from build123d import *


# Not quite as in the source:
# - a fillet or chamfer that OpenCascade refuses, or shapes differently, is made with other operations: its cross-section is extruded or revolved along the edge and cut away or added


with BuildPart() as f1:
    # F0 (on Front) → F1 (revolve)
    with BuildSketch(Plane.XZ):
        Polygon((-3.0760182999, 0), (0, 0), (0, 7.6753781177), (10.0012486801, 7.6753781177), (10.0012486801, 75.3582566977), (13.1937107071, 75.3582566977), (13.1937107071, 78.3602893353), (6.8093864247, 78.3602893353), (6.8093864247, 10.8100166544), (-3.0760182999, 10.8100166544), align=None)
    revolve(axis=Axis((-14.1970999539, 0, 39.5920351148), (0, 0, 1)))

    # F2: fillet of radius 5.08 on 1 edges, made by hand

    # F2_s1 → F2_t2 (revolve, cut)
    with BuildSketch(Plane.XZ):
        with BuildLine():
            ThreePointArc((13.1937107071, 75.3582566977), (11.3195166688, 77.544235524), (8.5581469182, 78.3602893353))
            Line((8.5581469182, 78.3602893353), (13.1937107071, 78.3602893353))
            Line((13.1937107071, 78.3602893353), (13.1937107071, 75.3582566977))
        make_face()
    revolve(axis=Axis((-14.1970999539, 0, 78.3602893353), (0, 0, 1)), mode=Mode.SUBTRACT)


solid = f1.part
Geometry check sheet. Reference: the model listing, model coordinates, mm. A direction names the side the tool comes from. Coordinates: 2 decimals unless noted, no trailing zeros. Order: outer loops, then holes, each group sorted by start corner. A loop starts at its lowest first (then second) coordinate and runs counter-clockwise, first axis right, second up. Notation, with made-up numbers: (45.5, 81.25) -> (80.5, 81.25) arc R24 ccw to (80.5, 91.25) -> close; hole circle Ø3 at (66, 24.25). An arc over 180 degrees is marked (long way). Use a Markdown table: item, result. Add a question column.
1. Cross-section at A-A (y = 0). Enter the section's corners in (x, z).
2. Go/stop test with flat-tipped pins: pin 1 Ø4 at (x, z) = (3, 49) entering from +Y; pin 2 Ø10 at (x, z) = (-12, 68.5) entering from +Y; pin 3 Ø1.5 at (x, z) = (-21, 44.5) entering from -Y. Record where each tip stops, or that it passes through.
3. Cross-section at B-B (z = 6). Enter the section's corners in (x, y).
4. Cross-section at C-C (z = 31). Enter the section's corners in (x, y), and give its area (3 significant figures).
5. Set-up check for faces 1 (the face through (-33.4, -14.724, 41.991)), 2 (the face through (-5, -9, 10.81)), 3 (the face through (-20.44, -9.4, 0)): record each of +Z, -Z, +X, -X, +Y, -Y from which the full face is reachable in a straight line by a thin tool's end or side.
6. Mould release check, pull along X, two halves, no side actions. Record for faces 4 (the face through (-23.02, -6.77, 5.33)), 5 (the face through (-24.2, -22.2, 75.358)), 6 (the face through (-28.38, 0.62, 3.89)): pulls with the +X half, pulls with the -X half, needs draft (parallel to the pull), parting line crosses it, or undercut.
7. Material ranges on L1, parallel to Y at x = -14, z = 61; L2, parallel to Z at x = -29.5, y = -14.5; L3, parallel to X at y = 0.5, z = 7, recorded low to high.
Filled sheet:
| question | item | result |
|---|---|---|
| 1 | outline | (-41.59, 75.36) -> (-38.4, 75.36) -> (-38.4, 7.68) -> (-28.39, 7.68) -> (-28.39, 0) -> (-25.32, 0) -> (-25.32, 10.81) -> (-35.2, 10.81) -> (-35.2, 78.36) -> (-36.95, 78.36) arc R5.08 ccw to start; (-3.08, 0) -> (0, 0) -> (0, 7.68) -> (10, 7.68) -> (10, 75.36) -> (13.19, 75.36) arc R5.08 ccw to (8.56, 78.36) -> (6.81, 78.36) -> (6.81, 10.81) -> (-3.08, 10.81) -> close |
| 2 | pin 1 | y = 18.83 |
| 2 | pin 2 | y = 24.2 |
| 2 | pin 3 | y = -23.43 |
| 3 | outline | circle Ø28.39 at (-14.2, 0); hole circle Ø22.24 at (-14.2, 0) |
| 4 | outline | circle Ø48.4 at (-14.2, 0); hole circle Ø42.01 at (-14.2, 0) |
| 4 | area | 453 mm2 |
| 5 | face 1 | -Z |
| 5 | face 2 | +Z |
| 5 | face 3 | -Z, +X, -X, +Y, -Y |
| 6 | face 4 | undercut |
| 6 | face 5 | needs draft |
| 6 | face 6 | parting line crosses it |
| 7 | L1 | -24.2 to -21.01, 21.01 to 24.2 |
| 7 | L2 | 7.68 to 78.36 |
| 7 | L3 | -28.39 to -25.31, -3.09 to -0.01 |
